Here's how the part is built. I have some questions about the finished solid (model axes, mm). Face numbers are marked on the shaded views. Coordinates: 2 decimals unless noted, no trailing zeros. Order: outer loops, then holes, each group sorted by start corner. A loop starts at its lowest first (then second) coordinate and runs counter-clockwise, first axis right, second up. Notation, with made-up numbers: M -31,-31 L 4,-31 A21 ccw 4,1 Z; hole C -6.75,27.25 d1. An arc over 180 degrees is marked long. Answer as CSV lines item,"result". Start each with the question number.
```python
from build123d import *

# Parameters (mm, degrees)
SKETCH1_R           = 39
SKETCH1_R_2         = 25
BOSS_EXTRUDE1_DEPTH = 10


with BuildPart() as part:
    # Sketch1 → Boss-Extrude1 (new body)
    # profile 1 of 20: a face of its own
    with BuildSketch(Plane.XY):
        Circle(SKETCH1_R)
        Circle(SKETCH1_R_2, mode=Mode.SUBTRACT)
    # profile 2 of 20: a face of its own
    with BuildSketch(Plane.XY):
        with BuildLine():
            ThreePointArc((-38.722045261, 4.647925426), (-37.806610372, 9.573933998), (-36.26719039, 14.341928085))
            Line((-36.26719039, 14.341928085), (-42.125470405, 15.825446064))
            Line((-42.125470405, 15.825446064), (-44.580325277, 6.131443405))
            Line((-44.580325277, 6.131443405), (-38.722045261, 4.647925426))
        make_face()
    # profile 3 of 20: a face of its own
    with BuildSketch(Plane.XY):
        with BuildLine():
            ThreePointArc((-35.114799123, 16.969115549), (-32.649492652, 21.330978167), (-29.645317542, 25.340780332))
            Line((-29.645317542, 25.340780332), (-34.704482287, 28.646097626))
            Line((-34.704482287, 28.646097626), (-40.173963868, 20.274432843))
            Line((-40.173963868, 20.274432843), (-35.114799123, 16.969115549))
        make_face()
    # profile 4 of 20: a face of its own
    with BuildSketch(Plane.XY):
        with BuildLine():
            ThreePointArc((-27.702319638, 27.451438699), (-23.954295795, 30.776479866), (-19.810914544, 33.593565826))
            Line((-19.810914544, 33.593565826), (-23.522725017, 38.36250002))
            Line((-23.522725017, 38.36250002), (-31.414130111, 32.220372893))
            Line((-31.414130111, 32.220372893), (-27.702319638, 27.451438699))
        make_face()
    # profile 5 of 20: a face of its own
    with BuildSketch(Plane.XY):
        with BuildLine():
            ThreePointArc((-17.287863974, 34.958972514), (-12.663279299, 36.886872426), (-7.829691557, 38.205967206))
            Line((-7.829691557, 38.205967206), (-9.791915499, 43.921730281))
            Line((-9.791915499, 43.921730281), (-19.250087916, 40.674735589))
            Line((-19.250087916, 40.674735589), (-17.287863974, 34.958972514))
        make_face()
    # profile 6 of 20: a face of its own
    with BuildSketch(Plane.XY):
        with BuildLine():
            Line((9.791915499, 43.921730281), (7.829691557, 38.205967206))
            ThreePointArc((7.829691557, 38.205967206), (12.663279299, 36.886872426), (17.287863974, 34.958972514))
            Line((17.287863974, 34.958972514), (19.250087916, 40.674735589))
            Line((19.250087916, 40.674735589), (9.791915499, 43.921730281))
        make_face()
    # profile 7 of 20: a face of its own
    with BuildSketch(Plane.XY):
        with BuildLine():
            Line((5, 44.72135955), (-5, 44.72135955))
            Line((-5, 44.72135955), (-5, 38.678159212))
            ThreePointArc((-5, 38.678159212), (0, 39), (5, 38.678159212))
            Line((5, 38.678159212), (5, 44.72135955))
        make_face()
    # profile 8 of 20: a face of its own
    with BuildSketch(Plane.XY):
        with BuildLine():
            Line((23.522725017, 38.36250002), (19.810914544, 33.593565826))
            ThreePointArc((19.810914544, 33.593565826), (23.954295795, 30.776479866), (27.702319638, 27.451438699))
            Line((27.702319638, 27.451438699), (31.414130111, 32.220372893))
            Line((31.414130111, 32.220372893), (23.522725017, 38.36250002))
        make_face()
    # profile 9 of 20: a face of its own
    with BuildSketch(Plane.XY):
        with BuildLine():
            Line((34.704482287, 28.646097626), (29.645317542, 25.340780332))
            ThreePointArc((29.645317542, 25.340780332), (32.649492652, 21.330978167), (35.114799123, 16.969115549))
            Line((35.114799123, 16.969115549), (40.173963868, 20.274432843))
            Line((40.173963868, 20.274432843), (34.704482287, 28.646097626))
        make_face()
    # profile 10 of 20: a face of its own
    with BuildSketch(Plane.XY):
        with BuildLine():
            Line((42.125470405, 15.825446064), (36.26719039, 14.341928085))
            ThreePointArc((36.26719039, 14.341928085), (37.806610372, 9.573933998), (38.722045261, 4.647925426))
            Line((38.722045261, 4.647925426), (44.580325277, 6.131443405))
            Line((44.580325277, 6.131443405), (42.125470405, 15.825446064))
        make_face()
    # profile 11 of 20: a face of its own
    with BuildSketch(Plane.XY):
        with BuildLine():
            Line((44.981510161, 1.289861865), (38.958950416, 1.788905393))
            ThreePointArc((38.958950416, 1.788905393), (38.989736253, 0.894688154), (39, 0))
            ThreePointArc((39, 0), (38.782683774, -4.111379241), (38.133156961, -8.176939537))
            Line((38.133156961, -8.176939537), (44.155716706, -8.675983065))
            Line((44.155716706, -8.675983065), (44.981510161, 1.289861865))
        make_face()
    # profile 12 of 20: a face of its own
    with BuildSketch(Plane.XY):
        with BuildLine():
            Line((42.963105331, -13.385498882), (37.428903653, -10.957972956))
            ThreePointArc((37.428903653, -10.957972956), (35.71515974, -15.666121561), (33.411949407, -20.115706223))
            Line((33.411949407, -20.115706223), (38.946151084, -22.543232149))
            Line((38.946151084, -22.543232149), (42.963105331, -13.385498882))
        make_face()
    # profile 13 of 20: a face of its own
    with BuildSketch(Plane.XY):
        with BuildLine():
            Line((36.288981397, -26.610333128), (31.842854411, -22.517384905))
            ThreePointArc((31.842854411, -22.517384905), (28.693232516, -26.413981293), (25.070038695, -29.874624012))
            Line((25.070038695, -29.874624012), (29.516165681, -33.967572235))
            Line((29.516165681, -33.967572235), (36.288981397, -26.610333128))
        make_face()
    # profile 14 of 20: a face of its own
    with BuildSketch(Plane.XY):
        with BuildLine():
            ThreePointArc((-38.133156961, -8.176939537), (-38.866795227, -3.220594473), (-38.958950416, 1.788905393))
            Line((-38.958950416, 1.788905393), (-44.981510161, 1.289861865))
            Line((-44.981510161, 1.289861865), (-44.155716706, -8.675983065))
            Line((-44.155716706, -8.675983065), (-38.133156961, -8.176939537))
        make_face()
    # profile 15 of 20: a face of its own
    with BuildSketch(Plane.XY):
        with BuildLine():
            ThreePointArc((-33.411949407, -20.115706223), (-35.71515974, -15.666121561), (-37.428903653, -10.957972956))
            Line((-37.428903653, -10.957972956), (-42.963105331, -13.385498882))
            Line((-42.963105331, -13.385498882), (-38.946151084, -22.543232149))
            Line((-38.946151084, -22.543232149), (-33.411949407, -20.115706223))
        make_face()
    # profile 16 of 20: a face of its own
    with BuildSketch(Plane.XY):
        with BuildLine():
            ThreePointArc((-25.070038695, -29.874624012), (-28.693232516, -26.413981293), (-31.842854411, -22.517384905))
            Line((-31.842854411, -22.517384905), (-36.288981397, -26.610333128))
            Line((-36.288981397, -26.610333128), (-29.516165681, -33.967572235))
            Line((-29.516165681, -33.967572235), (-25.070038695, -29.874624012))
        make_face()
    # profile 17 of 20: a face of its own
    with BuildSketch(Plane.XY):
        with BuildLine():
            ThreePointArc((-14.011400288, -36.396162737), (-18.561948328, -34.299476297), (-22.8061378, -31.636688806))
            Line((-22.8061378, -31.636688806), (-25.682383247, -36.951524877))
            Line((-25.682383247, -36.951524877), (-16.887645735, -41.710998808))
            Line((-16.887645735, -41.710998808), (-14.011400288, -36.396162737))
        make_face()
    # profile 18 of 20: a face of its own
    with BuildSketch(Plane.XY):
        with BuildLine():
            ThreePointArc((-1.434409251, -38.973612485), (-6.419189021, -38.468090833), (-11.298022285, -37.327666582))
            Line((-11.298022285, -37.327666582), (-12.292700369, -43.288445544))
            Line((-12.292700369, -43.288445544), (-2.429087335, -44.934391447))
            Line((-2.429087335, -44.934391447), (-1.434409251, -38.973612485))
        make_face()
    # profile 19 of 20: a face of its own
    with BuildSketch(Plane.XY):
        with BuildLine():
            Line((12.292700369, -43.288445544), (11.298022285, -37.327666582))
            ThreePointArc((11.298022285, -37.327666582), (6.419189021, -38.468090833), (1.434409251, -38.973612485))
            Line((1.434409251, -38.973612485), (2.429087335, -44.934391447))
            Line((2.429087335, -44.934391447), (12.292700369, -43.288445544))
        make_face()
    # profile 20 of 20: a face of its own
    with BuildSketch(Plane.XY):
        with BuildLine():
            Line((25.682383247, -36.951524877), (22.8061378, -31.636688806))
            ThreePointArc((22.8061378, -31.636688806), (18.561948328, -34.299476297), (14.011400288, -36.396162737))
            Line((14.011400288, -36.396162737), (16.887645735, -41.710998808))
            Line((16.887645735, -41.710998808), (25.682383247, -36.951524877))
        make_face()
    extrude(amount=BOSS_EXTRUDE1_DEPTH)


solid = part.part
```
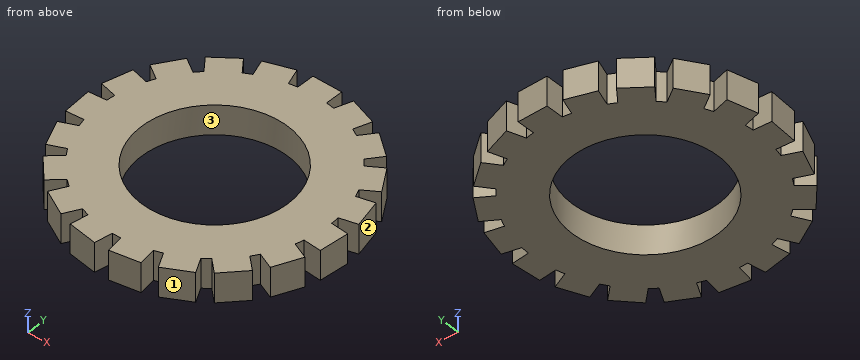
1) Will these pins go through, and if not, where does the flat tip stop? pin 1 Ø2 at (y, z) = (26, 3.5) entering from +X; pin 2 Ø2 at (x, y) = (-30, -24.5) entering from -Z; pin 3 Ø1.5 at (x, z) = (18.5, 2.5) entering from +Y; pin 4 Ø2 at (x, z) = (-32, 2) entering from -Y.
2) I need wall thicknesses on line 1 (Y direction, x = 0, z = 2.25); line 2 (X direction, y = 39, z = 9.25); line 3 (Y direction, x = -29.5, z = 9.25). Which ranges of each line are inside material? Lowest first, please. Write a range as [from, to].
3) Suppose I cut it at B-B on y = 0. Please give me the cut outline in (x, z), plus the area to 3 significant figures.
4) Suppose I cut it at A-A on x = 0. Please give me the cut outline in (y, z), plus the area to 3 significant figures.
5) If we mould it in two halves opening along Y, with no side actions, what happens to the marked faces 1, 2 and 3? For each: released by +Y, released by -Y, zero draft, split by the parting line, or undercut.
Output:
1,pin 1,"x = 37.09"
1,pin 2,"z = 0"
1,pin 3,"y = 41.19"
1,pin 4,"y = -32.36"
2,line 1,"[-39, -25], [25, 44.72]"
2,line 2,"[-18.68, -8.1], [-5, 5], [8.1, 18.68]"
2,line 3,"[-33.95, 25.51], [29.76, 33.71]"
3,outline,"M -44.87,0 L -25,0 L -25,10 L -44.87,10 Z; M 25,0 L 44.87,0 L 44.87,10 L 25,10 Z"
3,area,"397 mm²"
4,outline,"M -39,0 L -25,0 L -25,10 L -39,10 Z; M 25,0 L 44.72,0 L 44.72,10 L 25,10 Z"
4,area,"337 mm²"
5,face 1,"released by -Y"
5,face 2,"released by +Y"
5,face 3,"undercut"
